Autodesk Inventor part; units mm, degrees
ref_plane "작업 평면1" through (0, 30, 0) normal (0, -1, 0) x (1, 0, 0)
ref_plane "YZ Plane" through (0, 0, 0) normal (1, 0, 0) x (0, 1, 0)
ref_plane "XZ Plane" through (0, 0, 0) normal (0, 1, 0) x (-1, 0, 0)
sketch "스케치1" plane through (0, 0, 0) normal (0, 0, 1) x (1, 0, 0)
  line L0 (0, 0) -> (40, 0)
  line L1 (40, 0) -> (40, 60)
  line L2 (40, 60) -> (0, 60)
  line L3 (0, 60) -> (0, 0)
  line L4 (10, 5) -> (30, 5)
  line L5 (30, 5) -> (30, 55)
  line L6 (30, 55) -> (10, 55)
  line L7 (10, 55) -> (10, 5)
  point P0 (20, 55)
  point P1 (20, 60)
  point P2 (10, 30)
  point P3 (0, 30)
  dimension "d0" = 60
  dimension "d1" = 40
  dimension "d4" = 5
  dimension "d5" = 10
extrude "돌출1" add sketch "스케치1" along normal blind 20 contours L3 L2 L1 L0 | L7 L6 L5 L4
extrude "돌출2" cut sketch "스케치1" along normal blind 20 contours L7 L6 L5 L4
sketch "스케치2" plane through (0, 0, 0) normal (0, -1, 0) x (1, 0, 0)
  line L0 (10, 0) -> (10, 20)
  line L1 (0, 0) -> (40, 0)
  line L2 (40, 0) -> (40, 20)
  line L3 (0, 20) -> (40, 20)
  line L4 (0, 0) -> (0, 20)
  line L5 (30, 0) -> (30, 20)
  circle A0 centre (15, 10) radius 2.6
  circle A1 centre (25, 10) radius 2.6
  point P0 (10, 10)
  point P1 (20, 20)
  dimension "d11" = 5.2
  dimension "d12" = 5.2
  dimension "d13" = 10
  dimension "d14" = 5
extrude "돌출3" cut sketch "스케치2" against normal through all contours A0 | A1
ref_plane "작업 평면1" through (0, 30, 0) normal (0, -1, 0) x (1, 0, 0)
properties part number "다리 연결 부품"
Read the model definition and answer for the solid it produces. Units are mm, in the model's axes. A direction names the side the tool comes from. Coordinates: 2 decimals unless noted, no trailing zeros. Order: outer loops, then holes, each group sorted by start corner. A loop starts at its lowest first (then second) coordinate and runs counter-clockwise, first axis right, second up. Notation, with made-up numbers: (51.5, 84.5) -> (60.5, 84.5) arc R9 ccw to (60.5, 98.5) -> close; hole circle Ø4 at (65.5, 18.5). An arc over 180 degrees is marked (long way). Answer as a JSON object with one key per item and string values.
1) A cutting plane is placed at A-A, the plane x = 25. Determine the outline of the cut face in (y, z).
Model answer:
{"outline": "(0, 0) -> (5, 0) -> (5, 7.4) -> (0, 7.4) -> close; (0, 12.6) -> (5, 12.6) -> (5, 20) -> (0, 20) -> close; (55, 0) -> (60, 0) -> (60, 7.4) -> (55, 7.4) -> close; (55, 12.6) -> (60, 12.6) -> (60, 20) -> (55, 20) -> close"}
2) Each of these flat-tipped pins is pushed along its axis until it touches: pin 1 (6 mm diameter, centred on x = 24.5, z = 9, fed in from -Y); pin 2 (4.5 mm diameter, centred on x = 25, z = 10, fed in from +Y). Where does it stop, or does it pass through?
Model answer:
{"pin 1": "stops at y = 0", "pin 2": "passes through"}
3) A cutting plane is placed at B-B, the plane y = 52.5. Determine the outline of the cut face in (x, z), plus the area to 3 significant figures.
Model answer:
{"outline": "(0, 0) -> (10, 0) -> (10, 20) -> (0, 20) -> close; (30, 0) -> (40, 0) -> (40, 20) -> (30, 20) -> close", "area": "400 mm²"}
4) A cutting plane is placed at D-D, the plane x = 29. Determine the outline of the cut face in (y, z).
Model answer:
{"outline": "(0, 0) -> (5, 0) -> (5, 20) -> (0, 20) -> close; (55, 0) -> (60, 0) -> (60, 20) -> (55, 20) -> close"}
5) A tool of negligible diameter and unlimited length cuts with its end or side. For faces 1 (the face through (30, 30, 10)), 2 (the face through (17.4, 57.5, 9)), from which of +Z, -Z, +X, -X, +Y, -Y can it reach the whole face along a straight path? Write none if from no direction.
Model answer:
{"face 1": "+Z, -Z", "face 2": "+Y, -Y"}
6) A cutting plane is placed at C-C, the plane z = 10. Determine the outline of the cut face in (x, y), plus the area to 3 significant figures.
Model answer:
{"outline": "(0, 0) -> (12.4, 0) -> (12.4, 5) -> (10, 5) -> (10, 55) -> (12.4, 55) -> (12.4, 60) -> (0, 60) -> close; (17.6, 0) -> (22.4, 0) -> (22.4, 5) -> (17.6, 5) -> close; (17.6, 55) -> (22.4, 55) -> (22.4, 60) -> (17.6, 60) -> close; (27.6, 0) -> (40, 0) -> (40, 60) -> (27.6, 60) -> (27.6, 55) -> (30, 55) -> (30, 5) -> (27.6, 5) -> close", "area": "1,300 mm²"}
7) The mould has two halves that part along X. Classify faces 3 (the face through (20, 0, 10)), 4 (the face through (40, 30, 10)), 5 (the face through (24.44, 2.46, 7.46)): released by +X, released by -X, zero draft, split by the parting line, or undercut.
Model answer:
{"face 3": "zero draft", "face 4": "released by +X", "face 5": "undercut"}
8) Consider line 1 along Y through (x, z) = (15, 3.5); line 2 along Z through (x, y) = (15, 57.7); line 3 along X through (y, z) = (12.5, 18.5). Determine where each line is inside the solid, lowest interval first. Write a range as from..to.
Model answer:
{"line 1": "y = 0..5, 55..60", "line 2": "z = 0..7.4, 12.6..20", "line 3": "x = 0..10, 30..40"}
